Source: CAD feature listing. Evaluate the final solid. Frame: model axes, mm. A direction names the side the tool comes from. Round coordinates to 2 decimals unless told otherwise and drop trailing zeros. Loops run counter-clockwise (first coordinate to the right, second up) from the corner with the lowest first, then second, coordinate; pieces in that order, holes last. Notation, with made-up numbers: M 80.5,85 L 100.5,85 A22 ccw 100.5,111 Z; hole C -37.75,77 d6. An arc over 180 degrees is marked long. One line per item, written item: value.
from build123d import *

# Parameters (mm, degrees)
CHAMFER_SIZE = 3


with BuildPart() as part:
    # Sketch → Revolution (revolve)
    with BuildSketch(Plane.XZ):
        Polygon((0, 4), (0, 10.5), (2, 10.5), (2, 15), (4, 15), (4, 4), align=None)
    revolve(axis=Axis((0, 0, 0), (1, 0, 0)))

    # Chamfer
    chamfer_edges = [part.edges().sort_by_distance(p)[0] for p in [
        (4, 0, -4),
    ]]
    chamfer(chamfer_edges, length=CHAMFER_SIZE)


solid = part.part
1. Ray query, line 1 (Z direction, x = 0.55, y = 0); line 2 (X direction, y = 13.5, z = 0). Return the intervals inside material, ascending. Write a range as [from, to].
Report:
line 1: z = [-10.5, -4], [4, 10.5]
line 2: x = [2, 4]
2. Section query D-D (z = -7.5). Return the cut outline in (x, y), and give its area (3 significant figures).
Report:
outline: M 0,-7.35 L 2,-7.35 L 2,-12.99 L 4,-12.99 L 4,12.99 L 2,12.99 L 2,7.35 L 0,7.35 Z
area: 81.4 mm2
3. Section query A-A (y = 0). Return the cut outline in (x, z).
Report:
outline: M 0,-10.5 L 2,-10.5 L 2,-15 L 4,-15 L 4,-7 L 1,-4 L 0,-4 Z; M 0,4 L 1,4 L 4,7 L 4,15 L 2,15 L 2,10.5 L 0,10.5 Z
4. Pin query (flat end, axial travel): pin 1 (2 mm diameter, centred on x = 1.5, y = 9, fed in from +Z); pin 2 (1 mm diameter, centred on y = -8, z = -10, fed in from -X); pin 3 (13 mm diameter, centred on y = 0, z = 0, fed in from +X). Return the tip coordinate at first contact, or that it passes through.
Report:
pin 1: stops at z = 12.6
pin 2: stops at x = 2
pin 3: stops at x = 3.5
5. Reachability of faces 1 (the face through (2, -10.2, -3.1)), 2 (the face through (1.15, 4.05, -0.9)) from +Z, -Z, +X, -X, +Y, -Y: full face, straight path, thin tool, end or side. Return the list, or none.
Report:
face 1: -X
face 2: +X
6. Pull-direction query (Z, two-part tool) for faces 3 (the face through (0, 0, -5)), 4 (the face through (0.493, 3.905, -0.867)), 5 (the face through (1, -3.2, 10)); classes: released by +Z, released by -Z, zero draft, split by the parting line, or undercut.
Report:
face 3: zero draft
face 4: undercut
face 5: split by the parting line
7. Section query C-C (x = 2.35). Return the cut outline in (y, z).
Report:
outline: C 0,0 d30; hole C 0,0 d10.7
